Part model, mm, in its own coordinate system. A direction names the side the tool comes from. Give positions to 0.01 mm unless a question says otherwise; leave off trailing zeros. Write each loop counter-clockwise with the first axis right and the second up, starting at its lowest first coordinate (ties: lowest second). Pieces come first, ordered by that corner, then holes. Notation, with made-up numbers: M -8.75,-33.5 L 18.25,-33.5 A20 cw 18.25,-7.5 Z; hole C 86,-28 d5. An arc over 180 degrees is marked long. Use a Markdown table: item, result.
```python
from build123d import *

# Parameters (mm, degrees)
F0_W     = 69
F0_H     = 44
F1_DEPTH = 440
F3_DEPTH = 40
F5_DEPTH = 40


with BuildPart() as f1:
    # F0 (on Right) → F1 (new body)
    with BuildSketch(Plane.YZ):
        with Locations((-3.159018, -14.54166)):
            Rectangle(F0_W, F0_H)
    extrude(amount=F1_DEPTH)

    # F2 (on face) → F3 (join)
    with BuildSketch(Plane(origin=(0, 0, 0), x_dir=(0, -1, 0), z_dir=(-1, 0, 0))):
        with BuildLine():
            ThreePointArc((-16.340982, -4.54166), (-26.340982, -14.54166), (-16.340982, -24.54166))
            Line((-16.340982, -24.54166), (22.659018, -24.54166))
            ThreePointArc((22.659018, -24.54166), (32.659018, -14.54166), (22.659018, -4.54166))
            Line((22.659018, -4.54166), (-16.340982, -4.54166))
        make_face()
    extrude(amount=F3_DEPTH)

    # F4 (on face) → F5 (join)
    with BuildSketch(Plane.YZ.offset(440)):
        with BuildLine():
            ThreePointArc((16.340982, -24.54166), (26.340982, -14.54166), (16.340982, -4.54166))
            Line((16.340982, -4.54166), (-22.659018, -4.54166))
            ThreePointArc((-22.659018, -4.54166), (-32.659018, -14.54166), (-22.659018, -24.54166))
            Line((-22.659018, -24.54166), (16.340982, -24.54166))
        make_face()
    extrude(amount=F5_DEPTH)


solid = f1.part
```
1. Cut at B-B, the plane z = -13. Give the cut face in (x, y), then the cut area to 3 significant figures.
Findings below:
| item | result |
|---|---|
| outline | M -40,-32.54 L 0,-32.54 L 0,-37.66 L 440,-37.66 L 440,-32.54 L 480,-32.54 L 480,26.22 L 440,26.22 L 440,31.34 L 0,31.34 L 0,26.22 L -40,26.22 Z |
| area | 35,100 mm2 |
2. Drill centre lines: L1, parallel to X at y = 23, z = -7; L2, parallel to Z at x = 444, y = -11. Where is each one in solid material? Low to high.
Findings below:
| item | result |
|---|---|
| L1 | 0 to 440 |
| L2 | -24.54 to -4.54 |
3. Cut at A-A, the plane y = 3. Give the cut face in (x, z).
Findings below:
| item | result |
|---|---|
| outline | M -40,-24.54 L 0,-24.54 L 0,-36.54 L 440,-36.54 L 440,-24.54 L 480,-24.54 L 480,-4.54 L 440,-4.54 L 440,7.46 L 0,7.46 L 0,-4.54 L -40,-4.54 Z |
4. Drop a flat-ended pin along its axis: P1, Ø19.5, axis at x = 452, y = 3.5, coming from the -Z side. Give the stop position or say it passes through.
Findings below:
| item | result |
|---|---|
| P1 | z = -24.54 |
5. Tool access for faces 1 (the flat face through (460, -3, -4.542)), 2 (the flat face through (-20, -3, -24.542)), 3 (the cylindrical face through (459.72, 26.34, -14.76)), 4 (the cylindrical face through (-19.72, -32.657, -14.762)), 5 (the flat face through (-20, -3, -4.542)): list every direction of +Z, -Z, +X, -X, +Y, -Y with a clear straight run to the whole face (end or side of a thin tool).
Findings below:
| item | result |
|---|---|
| face 1 | +Z, +X, +Y, -Y |
| face 2 | -Z, -X, +Y, -Y |
| face 3 | +X, +Y |
| face 4 | -X, -Y |
| face 5 | +Z, -X, +Y, -Y |
